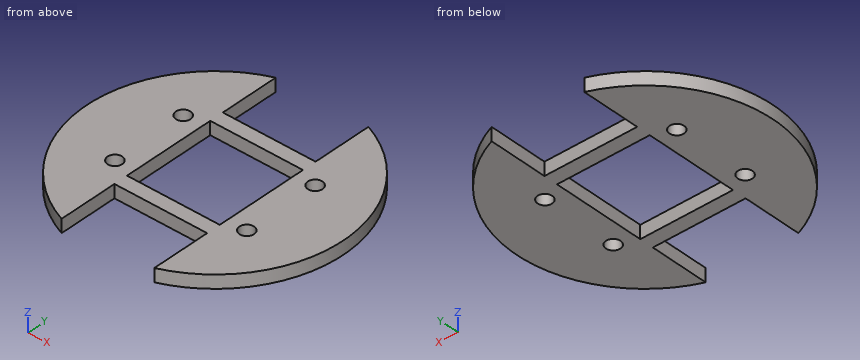
from build123d import *

# Parameters (mm, degrees)
SKETCH_1_R      = 1.65
SKETCH_1_W      = 21
SKETCH_1_H      = 21
EXTRUDE_1_DEPTH = 3


with BuildPart() as part:
    # 草图1 → 凸台-拉伸1 (new body)
    with BuildSketch(Plane.XY):
        with BuildLine():
            Line((10.5, -13.686215693), (10.5, -27.032387982))
            ThreePointArc((10.5, -27.032387982), (29, 0), (10.5, 27.032387982))
            Line((10.5, 27.032387982), (10.5, 13.686215693))
            Line((10.5, 13.686215693), (-10.5, 13.686215693))
            Line((-10.5, 13.686215693), (-10.5, 27.032387982))
            ThreePointArc((-10.5, 27.032387982), (-29, 0), (-10.5, -27.032387982))
            Line((-10.5, -27.032387982), (-10.5, -13.686215693))
            Line((-10.5, -13.686215693), (10.5, -13.686215693))
        make_face()
        with Locations((14.938938215, 8.625)):
            Circle(SKETCH_1_R, mode=Mode.SUBTRACT)
        with Locations((14.938938215, -8.625)):
            Circle(SKETCH_1_R, mode=Mode.SUBTRACT)
        with Locations((-14.938938215, -8.625)):
            Circle(SKETCH_1_R, mode=Mode.SUBTRACT)
        with Locations((-14.938938215, 8.625)):
            Circle(SKETCH_1_R, mode=Mode.SUBTRACT)
        Rectangle(SKETCH_1_W, SKETCH_1_H, mode=Mode.SUBTRACT)
    extrude(amount=EXTRUDE_1_DEPTH)


solid = part.part
Input: part model. Units: mm. Frame: model coordinates. Coordinates: 2 decimals unless noted, no trailing zeros. Loops run counter-clockwise (first coordinate to the right, second up) from the corner with the lowest first, then second, coordinate; pieces in that order, holes last. Notation, with made-up numbers: (-10, 9.5) - (37, 9.5) arc R22 cw to (37, 36.5) - close; hole circle Ø6 at (78, 35). An arc over 180 degrees is marked (long way). Answer in a Markdown table with one row per item. Add a question column.
Item 1: Section query B-B on y = -1.5. Return the cut outline in (x, z), then the cut area to 3 significant figures.
Item 2: Contact query for flat-ended pins moving along their axis: P1, Ø0.9, axis at y = 19.5, z = 2, coming from the -X side; P2, Ø0.9, axis at y = -21.5, z = 1.5, coming from the -X side; P3, Ø2, axis at x = -14.94, y = -8.62, coming from the -Z side; P4, Ø0.9, axis at y = 2, z = 2, coming from the +X side. Output: stop coordinate, or through.
Item 3: Section query A-A on x = -7. Return the cut outline in (y, z), then the cut area to 3 significant figures.
Item 4: Section query C-C on z = 1.5. Return the cut outline in (x, y) (3 decimals), then the cut area to 3 significant figures.
Item 5: Section query D-D on x = -21. Return the cut outline in (y, z), then the cut area to 3 significant figures.
Item 6: Line query: line 1 along Y through (x, z) = (5, 1.7); line 2 along X through (y, z) = (-9, 0.55); line 3 along Y through (x, z) = (-15.5, 0.9). Output: solid intervals per line, ascending. Write a range as [from, to].
Recorded:
| question | item | result |
|---|---|---|
| 1 | outline | (-28.96, 0) - (-10.5, 0) - (-10.5, 3) - (-28.96, 3) - close; (10.5, 0) - (28.96, 0) - (28.96, 3) - (10.5, 3) - close |
| 1 | area | 111 mm^2 |
| 2 | P1 | x = -21.87 |
| 2 | P2 | x = -19.95 |
| 2 | P3 | through |
| 2 | P4 | x = 28.96 |
| 3 | outline | (-13.69, 0) - (-10.5, 0) - (-10.5, 3) - (-13.69, 3) - close; (10.5, 0) - (13.69, 0) - (13.69, 3) - (10.5, 3) - close |
| 3 | area | 19.1 mm^2 |
| 4 | outline | (-10.5, -27.032) - (-10.5, -13.686) - (10.5, -13.686) - (10.5, -27.032) arc R29 ccw to (10.5, 27.032) - (10.5, 13.686) - (-10.5, 13.686) - (-10.5, 27.032) arc R29 ccw to start; hole circle Ø3.3 at (-14.939, -8.625); hole circle Ø3.3 at (-14.939, 8.625); hole (-10.5, -10.5) - (10.5, -10.5) - (10.5, 10.5) - (-10.5, 10.5) - close; hole circle Ø3.3 at (14.939, -8.625); hole circle Ø3.3 at (14.939, 8.625) |
| 4 | area | 1,550 mm^2 |
| 5 | outline | (-20, 0) - (20, 0) - (20, 3) - (-20, 3) - close |
| 5 | area | 120 mm^2 |
| 6 | line 1 | [-13.69, -10.5], [10.5, 13.69] |
| 6 | line 2 | [-27.57, -16.55], [-13.33, -10.5], [10.5, 13.33], [16.55, 27.57] |
| 6 | line 3 | [-24.51, -10.18], [-7.07, 7.07], [10.18, 24.51] |
